```python
from build123d import *

# Parameters (mm, degrees)
F1_DEPTH = 40
F2_R     = 19.99999
F3_R     = 5
F4_DEPTH = 25
F5_R     = 5
F6_DEPTH = 25


# Not quite as in the source:
# - a fillet or chamfer is up to 0.001 mm smaller than in the source, because OpenCascade refuses the exact size


with BuildPart() as f1:
    # F0 (on Front) → F1 (new body)
    with BuildSketch(Plane.XZ):
        Polygon((0, -10), (0, 0), (0, 20), (-20, 20), (-20, -20), (0, -20), (40, -20), (40, -10), align=None)
    extrude(amount=F1_DEPTH)

    # F2 (radius 20 in the source; OpenCascade refuses exactly that, so slightly less here)
    f2_edges = [f1.edges().sort_by_distance(p)[0] for p in [
        (40, -40, -15),
        (40, 0, -15),
    ]]
    fillet(f2_edges, radius=F2_R)

    # F3 (on face) → F4 (cut)
    with BuildSketch(Plane.XY.offset(-10)):
        with Locations((20, -20)):
            Circle(F3_R)
    extrude(amount=-F4_DEPTH, mode=Mode.SUBTRACT)

    # F5 (on face) → F6 (cut)
    with BuildSketch(Plane.YZ):
        with Locations((-20, 5)):
            Circle(F5_R)
    extrude(amount=-F6_DEPTH, mode=Mode.SUBTRACT)


solid = f1.part
```
Can you work these out from the model? Positions are in its coordinate system, mm. A direction names the side the tool comes from. Give positions to 0.01 mm unless a question says otherwise; leave off trailing zeros. Order: outer loops, then holes, each group sorted by start corner. A loop starts at its lowest first (then second) coordinate and runs counter-clockwise, first axis right, second up. Notation, with made-up numbers: (47.25, -40) - (69.25, -40) arc R30 cw to (69.25, -15) - close; hole circle Ø11 at (78.5, -10.75). An arc over 180 degrees is marked (long way). Use a Markdown table: item, result. Add a question column.
Q1. I'm going to push flat-ended pins straight in: pin 1 (16 mm diameter, centred on x = 20, y = -20, fed in from +Z); pin 2 (9 mm diameter, centred on y = -26.5, z = 10, fed in from +X); pin 3 (12 mm diameter, centred on x = -10.5, z = 15.5, fed in from +Y). Where does each tip first touch, or does it pass through?
Q2. On a 3-axis mill with a long thin cutter (end or side, diameter ignored), from which of +Z, -Z, +X, -X, +Y, -Y can I reach the whole of each face in a straight line? I mean faces 1 (the flat face through (16, -24, -10)), 2 (the flat face through (-10, -20, 20)). Say none if no direction works.
Q3. If we section it at C-C on x = -8: Write out the boundary of the cut face in (y, z).
Q4. Please list where these lines run through material, in increasing order: line 1 along Z through (x, y) = (-14, -20); line 2 along Y through (x, z) = (20, -14.5); line 3 along Z through (x, y) = (25.5, -11).
Q5. If we section it at B-B on y = -18: Write out the boundary of the cut face in (x, z).
Q6. If we mould it in two halves opening along Y, with no side actions, what happens to faces 3 (the cylindrical face through (34.297, -33.986, -14.93)), 4 (the flat face through (-20, -20, -4)), 5 (the cylindrical face through (-10, -25, 5))? For each: released by +Y, released by -Y, zero draft, split by the parting line, or undercut.
Q7. If we section it at D-D on y = -36: Write out the boundary of the cut face in (x, z).
Q8. If we section it at A-A on z = 5: Write out the boundary of the cut face in (x, y).
Answers follow:
| question | item | result |
|---|---|---|
| 1 | pin 1 | stops at z = -10 |
| 1 | pin 2 | stops at x = 0 |
| 1 | pin 3 | stops at y = 0 |
| 2 | face 1 | +Z, +X, +Y, -Y |
| 2 | face 2 | +Z, +X, -X, +Y, -Y |
| 3 | outline | (-40, -20) - (0, -20) - (0, 20) - (-40, 20) - close; hole circle Ø10 at (-20, 5) |
| 4 | line 1 | z = -20 to 0, 10 to 20 |
| 4 | line 2 | y = -40 to -25, -15 to 0 |
| 4 | line 3 | z = -20 to -10 |
| 5 | outline | (-20, -20) - (15.42, -20) - (15.42, -10) - (0, -10) - (0, 0.42) - (-20, 0.42) - close; (-20, 9.58) - (0, 9.58) - (0, 20) - (-20, 20) - close; (24.58, -20) - (39.9, -20) - (39.9, -10) - (24.58, -10) - close |
| 6 | face 3 | released by -Y |
| 6 | face 4 | zero draft |
| 6 | face 5 | undercut |
| 7 | outline | (-20, -20) - (32, -20) - (32, -10) - (0, -10) - (0, 20) - (-20, 20) - close |
| 8 | outline | (-20, -40) - (0, -40) - (0, -25) - (-20, -25) - close; (-20, -15) - (0, -15) - (0, 0) - (-20, 0) - close |
